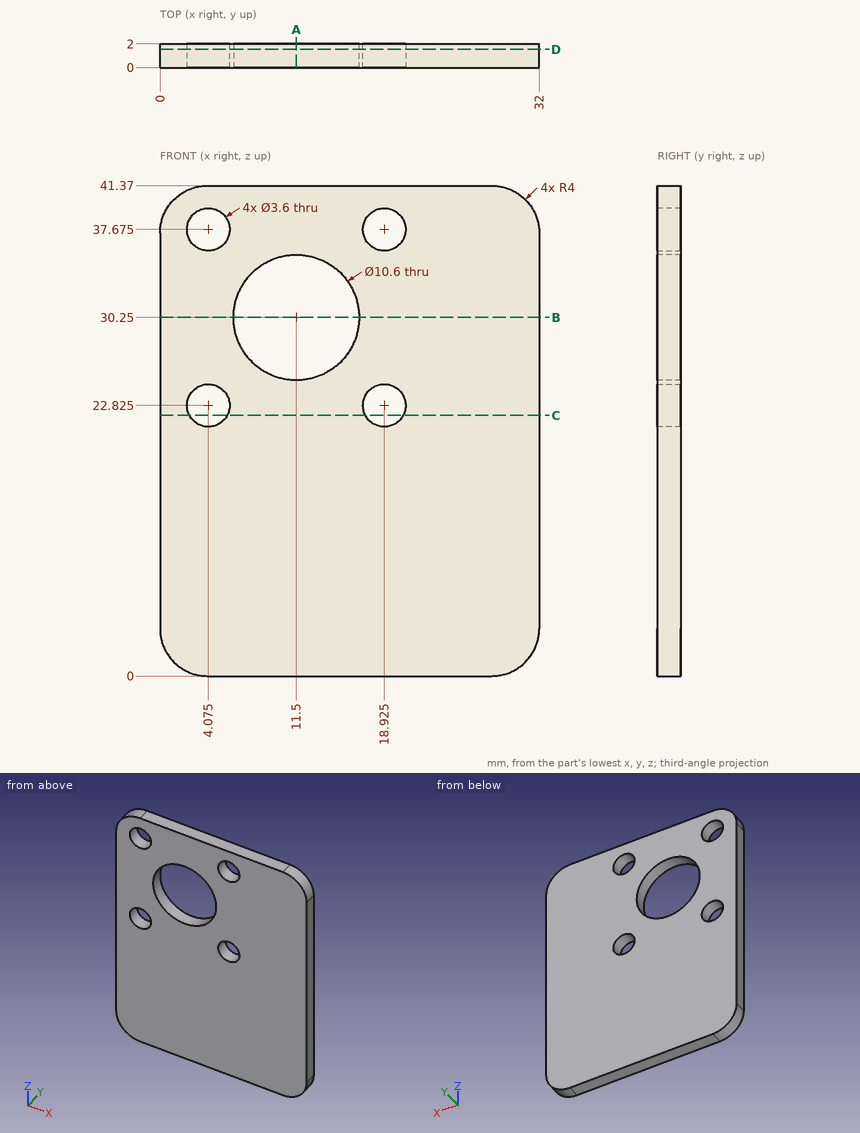
Design review of the part shown in the three views and the two pictorial views. Dimensions are in mm from the part's minimum x, y and z. Round coordinates to 2 decimals unless told otherwise and drop trailing zeros. Loops run counter-clockwise (first coordinate to the right, second up) from the corner with the lowest first, then second, coordinate; pieces in that order, holes last.
1) Consider section C-C on z = 22. State the section outline as (x, y) points (1 decimal).
Values follow:
outline: (0, 0) - (2.5, 0) - (2.5, 2) - (0, 2) - close; (5.7, 0) - (17.3, 0) - (17.3, 2) - (5.7, 2) - close; (20.5, 0) - (32, 0) - (32, 2) - (20.5, 2) - close
2) Consider section D-D on y = 1.55. Give the number of separate pieces and of enclosed holes in the cut face, then the cut area to 3 significant figures.
Values follow:
separate pieces: 1
enclosed holes: 5
area: 1,180 mm2
3) Consider section A-A on x = 11.5. State the section outline as (y, z) points.
Values follow:
outline: (0, 0) - (2, 0) - (2, 24.95) - (0, 24.95) - close; (0, 35.55) - (2, 35.55) - (2, 41.37) - (0, 41.37) - close
4) Consider section B-B on z = 30.25. State the section outline as (x, y) points.
Values follow:
outline: (0, 0) - (6.2, 0) - (6.2, 2) - (0, 2) - close; (16.8, 0) - (32, 0) - (32, 2) - (16.8, 2) - close
5) Wall thickness on line 1 along Z through (x, y) = (11.5, 1.1); line 2 along X through (y, z) = (1.95, 39) (1 decimal); line 3 along X through (y, z) = (1.3, 30.25): over which ranges is each line inside the solid? List them lowest first.
Values follow:
line 1: z = 0 to 24.95, 35.55 to 41.37
line 2: x = 0.3 to 2.9, 5.3 to 17.7, 20.1 to 31.7
line 3: x = 0 to 6.2, 16.8 to 32
